from build123d import *

# Parameters (mm, degrees)
CUT_EXTRUDE1_DEPTH  = 194.530714703
SKETCH7_W           = 174
SKETCH7_H           = 77.2
BOSS_EXTRUDE1_DEPTH = 2
CUT_EXTRUDE2_DEPTH  = 3
FILLET1_R           = 6
CHAMFER1_SIZE       = 6
CUT_EXTRUDE3_REACH  = 213.158


with BuildPart() as part:
    # Sweep1: sweep along a path in Sketch2
    with BuildLine(Plane(origin=(0, 0, 0), x_dir=(1, 0, 0), z_dir=(0, 1, 0))) as sweep1_path:
        Line((0, 0), (50, 0))
        Line((50, 0), (50, 180))
    # Sketch4 → Sweep1 (sweep)
    with BuildSketch(Plane(origin=(0, 0, 0), x_dir=(0, 0, -1), z_dir=(1, 0, 0))):
        Polygon((0, -40), (0, 40), (30, 48.038475773), (30, 50.538475773), (-2.5, 41.830127019), (-2.5, -41.830127019), (30, -50.538475773), (30, -48.038475773), align=None)
    sweep(path=sweep1_path.line, transition=Transition.RIGHT)

    # Sketch6 → Cut-Extrude1 (cut, through all)
    with BuildSketch(Plane.ZY.offset(-50)):
        with BuildLine():
            Line((-10, 28.4), (-170, 28.4))
            ThreePointArc((-170, 28.4), (-171.6, 30), (-170, 31.6))
            Line((-170, 31.6), (-10, 31.6))
            ThreePointArc((-10, 31.6), (-8.4, 30), (-10, 28.4))
        make_face()
        with BuildLine():
            Line((-10, -1.6), (-170, -1.6))
            ThreePointArc((-170, -1.6), (-171.6, 0), (-170, 1.6))
            Line((-170, 1.6), (-10, 1.6))
            ThreePointArc((-10, 1.6), (-8.4, 0), (-10, -1.6))
        make_face()
        with BuildLine():
            Line((-10, -31.6), (-170, -31.6))
            ThreePointArc((-170, -31.6), (-171.6, -30), (-170, -28.4))
            Line((-170, -28.4), (-10, -28.4))
            ThreePointArc((-10, -28.4), (-8.4, -30), (-10, -31.6))
        make_face()
        with BuildLine():
            Line((-10, -16.6), (-170, -16.6))
            ThreePointArc((-170, -16.6), (-171.6, -15), (-170, -13.4))
            Line((-170, -13.4), (-10, -13.4))
            ThreePointArc((-10, -13.4), (-8.4, -15), (-10, -16.6))
        make_face()
        with BuildLine():
            Line((-10, 13.4), (-170, 13.4))
            ThreePointArc((-170, 13.4), (-171.6, 15), (-170, 16.6))
            Line((-170, 16.6), (-10, 16.6))
            ThreePointArc((-10, 16.6), (-8.4, 15), (-10, 13.4))
        make_face()
    extrude(amount=-CUT_EXTRUDE1_DEPTH, mode=Mode.SUBTRACT)

    # Sketch7 → Boss-Extrude1 (add)
    with BuildSketch(Plane(origin=(52.5, 0, 0), x_dir=(0, 0, -1), z_dir=(1, 0, 0))):
        with Locations((90, 0)):
            Rectangle(SKETCH7_W, SKETCH7_H)
        with BuildLine():
            Line((170, -31.6), (10, -31.6))
            ThreePointArc((10, -31.6), (8.4, -30), (10, -28.4))
            Line((10, -28.4), (170, -28.4))
            ThreePointArc((170, -28.4), (171.6, -30), (170, -31.6))
        make_face(mode=Mode.SUBTRACT)
        with BuildLine():
            Line((170, -16.6), (10, -16.6))
            ThreePointArc((10, -16.6), (8.4, -15), (10, -13.4))
            Line((10, -13.4), (170, -13.4))
            ThreePointArc((170, -13.4), (171.6, -15), (170, -16.6))
        make_face(mode=Mode.SUBTRACT)
        with BuildLine():
            Line((10, 1.6), (170, 1.6))
            ThreePointArc((170, 1.6), (171.6, 0), (170, -1.6))
            Line((170, -1.6), (10, -1.6))
            ThreePointArc((10, -1.6), (8.4, 0), (10, 1.6))
        make_face(mode=Mode.SUBTRACT)
        with BuildLine():
            Line((170, 13.4), (10, 13.4))
            ThreePointArc((10, 13.4), (8.4, 15), (10, 16.6))
            Line((10, 16.6), (170, 16.6))
            ThreePointArc((170, 16.6), (171.6, 15), (170, 13.4))
        make_face(mode=Mode.SUBTRACT)
        with BuildLine():
            Line((170, 28.4), (10, 28.4))
            ThreePointArc((10, 28.4), (8.4, 30), (10, 31.6))
            Line((10, 31.6), (170, 31.6))
            ThreePointArc((170, 31.6), (171.6, 30), (170, 28.4))
        make_face(mode=Mode.SUBTRACT)
    extrude(amount=BOSS_EXTRUDE1_DEPTH)

    # Sketch9 → Cut-Extrude2 (cut)
    with BuildSketch(Plane.ZY.offset(-50)):
        with BuildLine():
            Line((-170, 33.6), (-10, 33.6))
            ThreePointArc((-10, 33.6), (-6.4, 30), (-10, 26.4))
            Line((-10, 26.4), (-170, 26.4))
            ThreePointArc((-170, 26.4), (-173.6, 30), (-170, 33.6))
        make_face()
        with BuildLine():
            Line((-170, 18.6), (-10, 18.6))
            ThreePointArc((-10, 18.6), (-6.4, 15), (-10, 11.4))
            Line((-10, 11.4), (-170, 11.4))
            ThreePointArc((-170, 11.4), (-173.6, 15), (-170, 18.6))
        make_face()
        with BuildLine():
            Line((-170, 3.6), (-10, 3.6))
            ThreePointArc((-10, 3.6), (-6.4, 0), (-10, -3.6))
            Line((-10, -3.6), (-170, -3.6))
            ThreePointArc((-170, -3.6), (-173.6, 0), (-170, 3.6))
        make_face()
        with BuildLine():
            Line((-170, -11.4), (-10, -11.4))
            ThreePointArc((-10, -11.4), (-6.4, -15), (-10, -18.6))
            Line((-10, -18.6), (-170, -18.6))
            ThreePointArc((-170, -18.6), (-173.6, -15), (-170, -11.4))
        make_face()
        with BuildLine():
            Line((-170, -26.4), (-10, -26.4))
            ThreePointArc((-10, -26.4), (-6.4, -30), (-10, -33.6))
            Line((-10, -33.6), (-170, -33.6))
            ThreePointArc((-170, -33.6), (-173.6, -30), (-170, -26.4))
        make_face()
    extrude(amount=-CUT_EXTRUDE2_DEPTH, mode=Mode.SUBTRACT)

    # Fillet1
    fillet1_edges = [part.edges().sort_by_distance(p)[0] for p in [
        (53.5, -38.6, -177),
        (53.5, 38.6, -177),
    ]]
    fillet(fillet1_edges, radius=FILLET1_R)

    # Chamfer1
    # the kernel refuses this chamfer: 6 mm, written as the material it adds along each edge
    with BuildSketch(Plane(origin=(52.5, -38.6, -3), x_dir=(-0.02749587661058908, 0, 0.9996219169112968), z_dir=(0, 1, 0))) as chamfer1_piece_1_section:
        Polygon((CHAMFER1_SIZE * 0.999621916911, CHAMFER1_SIZE * 0.0274958766106), (-CHAMFER1_SIZE * 0.0274958766106, CHAMFER1_SIZE * 0.999621916911), (0, 0), align=None)
    chamfer1_piece_1 = extrude(amount=77.2, mode=Mode.PRIVATE)
    chamfer1_piece_1 = split(chamfer1_piece_1, bisect_by=Plane(origin=(53.373608637, 0, 2.5), z_dir=(0, 0, -1)), keep=Keep.TOP, mode=Mode.PRIVATE)
    chamfer1_piece_1 = split(chamfer1_piece_1, bisect_by=Plane(origin=(54.5, 0, -0.51208469), z_dir=(-1, 0, 0)), keep=Keep.TOP, mode=Mode.PRIVATE)
    add(chamfer1_piece_1)

    # Sketch10 → Cut-Extrude3 (cut, up to next)
    with BuildSketch(Plane(origin=(13.974364905, 52.15303983, 0), x_dir=(0.9659258262890679, -0.25881904510252257, 0), z_dir=(0.2588190451025226, 0.9659258262890679, 0)), mode=Mode.PRIVATE) as cut_extrude3_sk1:
        with BuildLine():
            Line((14.538196485, 170), (14.538196485, 40))
            ThreePointArc((14.538196485, 40), (12.938196485, 38.4), (11.338196485, 40))
            Line((11.338196485, 40), (11.338196485, 170))
            ThreePointArc((11.338196485, 170), (12.938196485, 171.6), (14.538196485, 170))
        make_face()
    cut_extrude3_tool1 = extrude(cut_extrude3_sk1.sketch, amount=-CUT_EXTRUDE3_REACH, mode=Mode.PRIVATE) & part.part
    # Sketch10 → Cut-Extrude3 (cut, up to next)
    with BuildSketch(Plane(origin=(13.974364905, 52.15303983, 0), x_dir=(0.9659258262890679, -0.25881904510252257, 0), z_dir=(0.2588190451025226, 0.9659258262890679, 0)), mode=Mode.PRIVATE) as cut_extrude3_sk2:
        with BuildLine():
            Line((31.538196485, 170), (31.538196485, 40))
            ThreePointArc((31.538196485, 40), (29.938196485, 38.4), (28.338196485, 40))
            Line((28.338196485, 40), (28.338196485, 170))
            ThreePointArc((28.338196485, 170), (29.938196485, 171.6), (31.538196485, 170))
        make_face()
    cut_extrude3_tool2 = extrude(cut_extrude3_sk2.sketch, amount=-CUT_EXTRUDE3_REACH, mode=Mode.PRIVATE) & part.part
    cut_extrude3_1 = cut_extrude3_tool1.solids().sort_by_distance((26.471703, 48.804388, -105))[0]
    add(cut_extrude3_1, mode=Mode.SUBTRACT)
    cut_extrude3_2 = cut_extrude3_tool2.solids().sort_by_distance((42.892442, 44.404464, -105))[0]
    add(cut_extrude3_2, mode=Mode.SUBTRACT)
    cut_extrude3 = cut_extrude3_1 + cut_extrude3_2  # Cut-Extrude3 as one shape, for the pattern or mirror that repeats it

    # Mirror1: Cut-Extrude3 across plane
    add(cut_extrude3.mirror(Plane.ZX), mode=Mode.SUBTRACT)


solid = part.part
The listing builds one solid part. Answer for the finished solid, in the listing's coordinates (mm). A direction names the side the tool comes from. Round coordinates to 2 decimals unless told otherwise and drop trailing zeros. Write each loop counter-clockwise with the first axis right and the second up, starting at its lowest first coordinate (ties: lowest second). Pieces come first, ordered by that corner, then holes. Notation, with made-up numbers: M -37.5,-23 L 12.5,-23 A16 ccw 12.5,-1 Z; hole C 26.25,65 d9. An arc over 180 degrees is marked long. Write each question's results on one line, items separated by ' | '. Start each with the question number.
Item 1: A cutting plane is placed at B-B on y = -20.5. Write down the section's boundary in (x, z), and give its area (3 significant figures).
Item 2: A cutting plane is placed at C-C on x = 35. Write down the section's boundary in (y, z).
Item 3: For faces 1 (the face through (50, 8, -91)), 2 (the face through (53, 32, -89)), 3 (the face through (36.478, -46.123, -90.028)), determine the directions among +Z, -Z, +X, -X, +Y, -Y from which every point of the face is accessible in a straight line to the end or side of a thin tool.
Item 4: Straight lines are drawn through the part: L1, parallel to X at y = -35, z = -102.5; L2, parallel to X at y = -32, z = -29; L3, parallel to Y at x = 22, z = -53. For each, find the intervals that lie inside material, in ascending order. Write a range as [from, to].
Item 5: A cutting plane is placed at D-D on y = 36.5. Write down the section's boundary in (x, z).
Item 6: Flat-ended cylindrical pins translate along their axes: pin 1 Ø1.5 at (x, z) = (51, -115.5) entering from -Y; pin 2 Ø4 at (y, z) = (35.5, -158) entering from -X; pin 3 Ø12 at (x, z) = (23, -37) entering from -Y; pin 4 Ø10 at (x, z) = (13.5, -43.5) entering from +Y. Find the tip coordinate at first contact, or state that the pin passes through.
Item 7: A cutting plane is placed at A-A on z = -82.5. State how many separate pieces and enclosed holes the cut face has, and give its area (3 significant figures).
Item 8: For a pull along Y with two mould halves and no side action, classify faces 4 (the face through (53.514, -36.889, -175.196)), 5 (the face through (51.5, -14.9, -6.4)), 6 (the face through (52.5, 40, -116)), 7 (the face through (20.78, 45.28, -10.37)) as pulls with the +Y half, pulls with the -Y half, needs draft (parallel to the pull), parting line crosses it, or undercut.
Check sheet entries:
1) outline: M 0,0 L 50,0 L 50,-180 L 52.5,-180 L 52.5,-177 L 54.5,-177 L 54.5,1 L 53,2.5 L 0,2.5 Z | area: 939 mm²
2) outline: M -46.52,-180 L -44.02,-180 L -44.02,-15 L -40,0 L 40,0 L 44.02,-15 L 44.02,-180 L 46.52,-180 L 46.52,-15 L 41.83,2.5 L -41.83,2.5 L -46.52,-15 Z
3) face 1: -Z, -X | face 2: -X | face 3: +Z, -Z, +X, -Y
4) L1: [50, 54.5] | L2: [53, 54.5] | L3: [-50, -47.5], [47.5, 50]
5) outline: M 0,0 L 50,0 L 50,-180 L 52.5,-180 L 52.5,-175.56 L 54.5,-175.56 L 54.5,1 L 53,2.5 L 0,2.5 Z
6) pin 1: y = -42.43 | pin 2: x = 50 | pin 3: y = -50.54 | pin 4: through
7) separate pieces: 10 | enclosed holes: 0 | area: 352 mm²
8) face 4: pulls with the -Y half | face 5: undercut | face 6: needs draft | face 7: pulls with the +Y half
